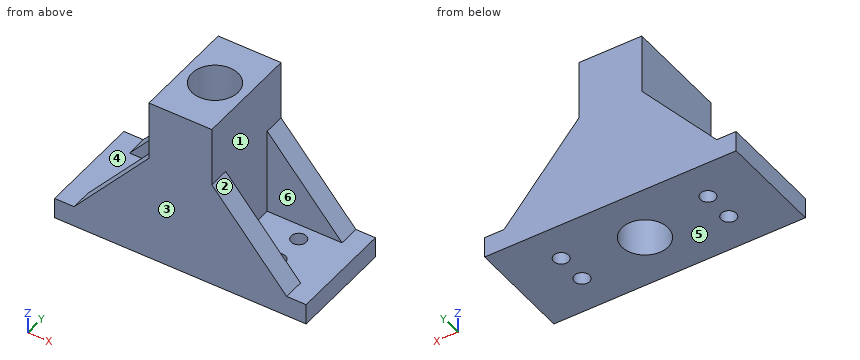
from build123d import *

# Parameters (mm, degrees)
SKETCH_1_W               = 40
SKETCH_1_H               = 15
EXTRUDE_1_DEPTH          = 5
SKETCH_2_R               = 5.5
SKETCH_2_R_2             = 1.8
CUT_EXTRUDE_1_DEPTH      = 5
SKETCH_3_W               = 15
SKETCH_3_H               = 15
SKETCH_3_R               = 5.05
EXTRUDE_2_DEPTH          = 25
SKETCH_4_R               = 5.5
CUT_EXTRUDE_2_DEPTH      = 31
SKETCH_5_W               = 10
SKETCH_5_H               = 15
EXTRUDE_3_DEPTH          = 5
SKETCH_6_R               = 1.8
CUT_EXTRUDE_3_DEPTH      = 5
SKETCH_7_W               = 60
SKETCH_7_H               = 5
EXTRUDE_4_DEPTH          = 5
SKETCH_8_W               = 15
SKETCH_8_H               = 5
EXTRUDE_5_DEPTH          = 25
RIB_1_REACH              = 51.244
SKETCH_9_WALL_W          = 127.83111072
SKETCH_9_WALL_H          = 5
MIRROR_2_COPY_1_REACH    = 51.244
MIRROR_2_COPY_1_SKETCH_W = 127.83111072
MIRROR_2_COPY_1_SKETCH_H = 5
SKETCH_11_R              = 1.8
EXTRUDE_6_DEPTH          = 5
SKETCH_12_R              = 1.8
CUT_EXTRUDE_4_DEPTH      = 5
SKETCH_13_W              = 15
SKETCH_13_H              = 25
SKETCH_13_R              = 5.5
EXTRUDE_7_DEPTH          = 10


with BuildPart() as part:
    # 草图1 → 凸台-拉伸1 (new body)
    with BuildSketch(Plane.XY):
        Rectangle(SKETCH_1_W, SKETCH_1_H)
    extrude(amount=EXTRUDE_1_DEPTH)

    # 草图2 → 切除-拉伸1 (cut)
    with BuildSketch(Plane.XY.offset(5)):
        Circle(SKETCH_2_R)
        with Locations((-12, 0)):
            Circle(SKETCH_2_R_2)
        with Locations(Location((12, 0, 0), (0, 0, 180))):
            Circle(SKETCH_2_R_2)
    extrude(amount=-CUT_EXTRUDE_1_DEPTH, mode=Mode.SUBTRACT)

    # 草图3 → 凸台-拉伸2 (add)
    with BuildSketch(Plane.XY.offset(5)):
        Rectangle(SKETCH_3_W, SKETCH_3_H)
        Circle(SKETCH_3_R, mode=Mode.SUBTRACT)
    extrude(amount=EXTRUDE_2_DEPTH)

    # 草图4 → 切除-拉伸2 (cut)
    with BuildSketch(Plane(origin=(0, 0, 5), x_dir=(-1, 0, 0), z_dir=(0, 0, -1))):
        with Locations(Location((0, 0, 0), (0, 0, 180))):
            Circle(SKETCH_4_R)
    extrude(amount=-CUT_EXTRUDE_2_DEPTH, mode=Mode.SUBTRACT)

    # 草图5 → 凸台-拉伸3 (add)
    with BuildSketch(Plane.XY.offset(5)):
        with Locations((-25, 0)):
            Rectangle(SKETCH_5_W, SKETCH_5_H)
        with Locations((25, 0)):
            Rectangle(SKETCH_5_W, SKETCH_5_H)
    extrude(amount=-EXTRUDE_3_DEPTH)

    # 草图6 → 切除-拉伸3 (cut)
    with BuildSketch(Plane.XY.offset(5)):
        with Locations((-24, 0)):
            Circle(SKETCH_6_R)
        with Locations(Location((24, 0, 0), (0, 0, 180))):
            Circle(SKETCH_6_R)
    extrude(amount=-CUT_EXTRUDE_3_DEPTH, mode=Mode.SUBTRACT)

    # 草图7 → 凸台-拉伸4 (add)
    with BuildSketch(Plane.XY.offset(5)):
        with Locations((0, 10)):
            Rectangle(SKETCH_7_W, SKETCH_7_H)
        with Locations((0, -10)):
            Rectangle(SKETCH_7_W, SKETCH_7_H)
    extrude(amount=-EXTRUDE_4_DEPTH)

    # 草图8 → 凸台-拉伸5 (add)
    with BuildSketch(Plane.XY.offset(5)):
        with Locations((0, 10)):
            Rectangle(SKETCH_8_W, SKETCH_8_H)
        with Locations((0, -10)):
            Rectangle(SKETCH_8_W, SKETCH_8_H)
    extrude(amount=EXTRUDE_5_DEPTH)

    # 草图9 wall → 筋1 (add, up to next)
    with BuildSketch(Plane(origin=(-16.427615827, 12.5, 15.353801199), x_dir=(0.653020400469, 0, 0.75734031754), z_dir=(0.75734031754, 0, -0.653020400469)), mode=Mode.PRIVATE) as rib_1_sk1:
        with Locations((0, 2.5)):
            Rectangle(SKETCH_9_WALL_W, SKETCH_9_WALL_H)
    rib_1_tool1 = extrude(rib_1_sk1.sketch, amount=RIB_1_REACH, mode=Mode.PRIVATE) - part.part
    rib_1 = rib_1_tool1.solids().sort_by_distance((-16.427615827, 12.5, 15.353801199))[0]
    add(rib_1)

    # 镜向1: 筋1 across plane
    add(rib_1.mirror(Plane.ZX))

    # 镜向2: 筋1 across plane
    add(rib_1.mirror(Plane.ZY))

    # 镜向2 copy 1 sketch → 镜向2 copy 1 (add, up to next)
    with BuildSketch(Plane(origin=(16.427615827, -12.5, 15.353801199), x_dir=(-0.653020400469, 0, 0.75734031754), z_dir=(-0.75734031754, 0, -0.653020400469)), mode=Mode.PRIVATE) as mirror_2_copy_1_sk1:
        with Locations((0, 2.5)):
            Rectangle(MIRROR_2_COPY_1_SKETCH_W, MIRROR_2_COPY_1_SKETCH_H)
    mirror_2_copy_1_tool1 = extrude(mirror_2_copy_1_sk1.sketch, amount=MIRROR_2_COPY_1_REACH, mode=Mode.PRIVATE) - part.part
    add(mirror_2_copy_1_tool1.solids().sort_by_distance((16.427615827, -12.5, 15.353801199))[0])

    # 草图11 → 凸台-拉伸6 (add)
    with BuildSketch(Plane.XY.offset(5)):
        with Locations((-24, 0)):
            Circle(SKETCH_11_R)
        with Locations((-12, 0)):
            Circle(SKETCH_11_R)
        with Locations((12, 0)):
            Circle(SKETCH_11_R)
        with Locations((24, 0)):
            Circle(SKETCH_11_R)
    extrude(amount=-EXTRUDE_6_DEPTH)

    # 草图12 → 切除-拉伸4 (cut)
    with BuildSketch(Plane.XY.offset(5)):
        with Locations((-17.5, 3.75)):
            Circle(SKETCH_12_R)
        with Locations(Location((-17.5, -3.75, 0), (0, 0, 180))):
            Circle(SKETCH_12_R)
        with Locations((17.5, -3.75)):
            Circle(SKETCH_12_R)
        with Locations(Location((17.5, 3.75, 0), (0, 0, 180))):
            Circle(SKETCH_12_R)
    extrude(amount=-CUT_EXTRUDE_4_DEPTH, mode=Mode.SUBTRACT)

    # 草图13 → 凸台-拉伸7 (add)
    with BuildSketch(Plane.XY.offset(30)):
        Rectangle(SKETCH_13_W, SKETCH_13_H)
        Circle(SKETCH_13_R, mode=Mode.SUBTRACT)
    extrude(amount=EXTRUDE_7_DEPTH)


solid = part.part
Read the model definition and answer for the solid it produces. Units are mm, in the model's axes. Face numbers are marked on the shaded views. A direction names the side the tool comes from. Coordinates: 2 decimals unless noted, no trailing zeros. Write each loop counter-clockwise with the first axis right and the second up, starting at its lowest first coordinate (ties: lowest second). Pieces come first, ordered by that corner, then holes. Notation, with made-up numbers: M 27,38 L 53,38 A13 ccw 53,49 Z; hole C -31.75,69.25 d9. An arc over 180 degrees is marked long. Use a Markdown table: item, result.
Q1. The part is cut by section A-A, the plane x = 0. Write down the section's boundary in (y, z).
Answer block:
| item | result |
|---|---|
| outline | M -12.5,0 L -5.5,0 L -5.5,40 L -12.5,40 Z; M 5.5,0 L 12.5,0 L 12.5,40 L 5.5,40 Z |
Q2. Straight lines are drawn through the part: L1, parallel to Y at x = -17.5, z = 3.65; L2, parallel to X at y = 0, z = 33; L3, parallel to Y at x = 0, z = 34.5. For each, find the intervals that lie inside material, in ascending order. Write a range as [from, to].
Answer block:
| item | result |
|---|---|
| L1 | y = [-12.5, -5.55], [-1.95, 1.95], [5.55, 12.5] |
| L2 | x = [-7.5, -5.5], [5.5, 7.5] |
| L3 | y = [-12.5, -5.5], [5.5, 12.5] |
Q3. Which of the six approach directions +Z, -Z, +X, -X, +Y, -Y give full straight-line access (tool end or side, diameter ignored) to the marked faces 4, 5 and 6?
Answer block:
| item | result |
|---|---|
| face 4 | +Z, -X |
| face 5 | -Z, +X, -X, +Y, -Y |
| face 6 | +Z, +X |
Q4. Determine the mould class of the marked faces 1, 2 and 3 for opening direction Y: released by +Y, released by -Y, zero draft, split by the parting line, or undercut.
Answer block:
| item | result |
|---|---|
| face 1 | undercut |
| face 2 | zero draft |
| face 3 | released by -Y |
Q5. The part is cut by section B-B, the plane y = 0. Write down the section's boundary in (x, z).
Answer block:
| item | result |
|---|---|
| outline | M -30,0 L -5.5,0 L -5.5,40 L -7.5,40 L -7.5,5 L -30,5 Z; M 5.5,0 L 30,0 L 30,5 L 7.5,5 L 7.5,40 L 5.5,40 Z |
Q6. Each of these flat-tipped pins is pushed along its axis until it touches: pin 1 Ø3 at (y, z) = (9.5, 21.5) entering from +X; pin 2 Ø7.5 at (y, z) = (-4, 27.5) entering from +X; pin 3 Ø9 at (x, z) = (-14, 19) entering from +Y; pin 4 Ø4 at (x, y) = (17.5, -3.75) entering from +Z. Where does it stop, or does it pass through?
Answer block:
| item | result |
|---|---|
| pin 1 | stops at x = 12.42 |
| pin 2 | stops at x = 7.5 |
| pin 3 | stops at y = 12.5 |
| pin 4 | stops at z = 5 |
Q7. The part is cut by section D-D, the plane z = 8. Write down the section's boundary in (x, y).
Answer block:
| item | result |
|---|---|
| outline | M -22.77,-12.5 L 22.77,-12.5 L 22.77,-7.5 L 7.5,-7.5 L 7.5,7.5 L 22.77,7.5 L 22.77,12.5 L -22.77,12.5 L -22.77,7.5 L -7.5,7.5 L -7.5,-7.5 L -22.77,-7.5 Z; hole C 0,0 d11 |
Q8. The part is cut by section C-C, the plane x = 17.5. Write down the section's boundary in (y, z), then the cut area to 3 significant figures.
Answer block:
| item | result |
|---|---|
| outline | M -12.5,0 L -5.55,0 L -5.55,5 L -7.5,5 L -7.5,14.11 L -12.5,14.11 Z; M -1.95,0 L 1.95,0 L 1.95,5 L -1.95,5 Z; M 5.55,0 L 12.5,0 L 12.5,14.11 L 7.5,14.11 L 7.5,5 L 5.55,5 Z |
| area | 180 mm2 |
